Read the model definition and answer for the solid it produces. Units are mm, in the model's axes. Coordinates: 2 decimals unless noted, no trailing zeros. Loops run counter-clockwise (first coordinate to the right, second up) from the corner with the lowest first, then second, coordinate; pieces in that order, holes last.
Solid Edge part; units mm, degrees
sketch "Sketch1" plane through (0, 0, 0) normal (0, 0, 1) x (1, 0, 0)
  line L0 (0.7047, -78.9141) -> (34.7047, -78.9141)
  line L1 (34.7047, -78.9141) -> (34.7047, -18.9141)
  line L2 (34.7047, -18.9141) -> (0.7047, -18.9141)
  line L3 (0.7047, -18.9141) -> (0.7047, -78.9141)
extrude "Protrusion1" add sketch "Sketch1" along normal blind 5
fillet "Round_1" radius 2 12 edges at (0.7047, -48.9141, 0) (17.7047, -78.9141, 0) (34.7047, -48.9141, 0) (17.7047, -18.9141, 0) (34.7047, -48.9141, 5) (17.7047, -78.9141, 5) (0.7047, -48.9141, 5) (17.7047, -18.9141, 5) (0.7047, -18.9141, 2.5) (0.7047, -78.9141, 2.5) (34.7047, -78.9141, 2.5) (34.7047, -18.9141, 2.5)
properties material "Zinc"
Q1. A cutting plane is placed at A-A (y = -56). Give the vertices of the cut face in (x, z).
Findings below:
outline: (0.7, 2) arc R2 ccw to (2.7, 0) - (32.7, 0) arc R2 ccw to (34.7, 2) - (34.7, 3) arc R2 ccw to (32.7, 5) - (2.7, 5) arc R2 ccw to (0.7, 3) - close
Q2. Straight lines are drawn through the part: probe 1 along Y at (x, z) = (4.5, 1.9); probe 2 along X at (y, z) = (-32, 3.1); probe 3 along Y at (x, z) = (18.5, 4.1). For each, find the intervals that lie inside material, in ascending order.
Findings below:
probe 1: y = -78.91 to -18.92
probe 2: x = 0.71 to 34.7
probe 3: y = -78.58 to -19.24
Q3. A cutting plane is placed at B-B (z = 0.6). Give the vertices of the cut face in (x, y).
Findings below:
outline: (1.28, -76.91) arc R1.43 ccw to (2.7, -78.34) - (32.7, -78.34) arc R1.43 ccw to (34.13, -76.91) - (34.13, -20.91) arc R1.43 ccw to (32.7, -19.49) - (2.7, -19.49) arc R1.43 ccw to (1.28, -20.91) - close
